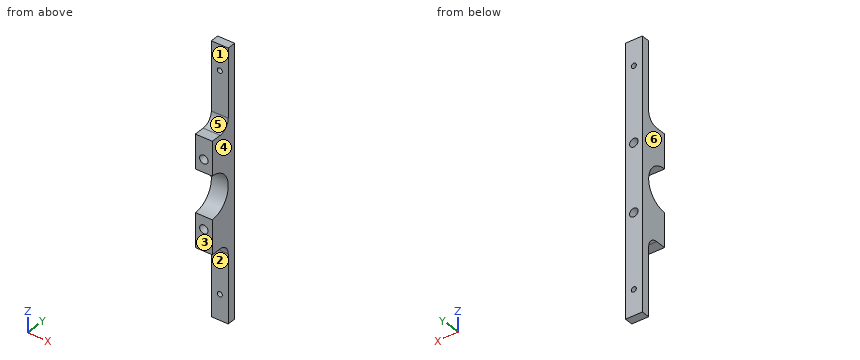
from build123d import *

# Parameters (mm, degrees)
BOSS_EXTRUDE1_DEPTH     = 10
CUT_EXTRUDE1_DEPTH      = 81.605520903
CUT_EXTRUDE1_DEPTH_BACK = 81.605520903
SKETCH2_R               = 1.5
SKETCH2_R_2             = 2.5
FILLET1_R               = 6.35


with BuildPart() as part:
    # Sketch1 → Boss-Extrude1 (new body)
    with BuildSketch(Plane(origin=(0, 0, 0), x_dir=(0, 0, -1), z_dir=(1, 0, 0))):
        with BuildLine():
            Line((-79, 12.5), (-32.5, 12.5))
            Line((-32.5, 12.5), (-32.5, 0))
            Line((-32.5, 0), (-12.5, 0))
            ThreePointArc((-12.5, 0), (0, 12.5), (12.5, 0))
            Line((12.5, 0), (32.5, 0))
            Line((32.5, 0), (32.5, 12.5))
            Line((32.5, 12.5), (79, 12.5))
            Line((79, 12.5), (79, 17.5))
            Line((79, 17.5), (-79, 17.5))
            Line((-79, 17.5), (-79, 12.5))
        make_face()
    extrude(amount=BOSS_EXTRUDE1_DEPTH)

    # Sketch2 → Cut-Extrude1 (cut, two sides: drawn at the far end of the back side and taken through both)
    with BuildSketch(Plane.XZ.offset(-12.5).offset(-CUT_EXTRUDE1_DEPTH_BACK)):
        with Locations(Location((5, 64, 0), (0, 0, 270))):
            Circle(SKETCH2_R)
        with Locations(Location((5, -64, 0), (0, 0, 90))):
            Circle(SKETCH2_R)
        with Locations(Location((5, 20, 0), (0, 0, 270))):
            Circle(SKETCH2_R_2)
        with Locations(Location((5, -20, 0), (0, 0, 90))):
            Circle(SKETCH2_R_2)
    extrude(amount=CUT_EXTRUDE1_DEPTH + CUT_EXTRUDE1_DEPTH_BACK, mode=Mode.SUBTRACT)

    # Fillet1
    fillet1_edges = [part.edges().sort_by_distance(p)[0] for p in [
        (5, 12.5, 32.5),
        (5, 12.5, -32.5),
    ]]
    fillet(fillet1_edges, radius=FILLET1_R)


solid = part.part
Geometry check sheet. Reference: the model listing, model coordinates, mm. Face numbers are marked on the shaded views. A direction names the side the tool comes from. Coordinates: 2 decimals unless noted, no trailing zeros. Order: outer loops, then holes, each group sorted by start corner. A loop starts at its lowest first (then second) coordinate and runs counter-clockwise, first axis right, second up. Notation, with made-up numbers: (31, -19) -> (72, -19) arc R24 cw to (72, 10) -> close; hole circle Ø6 at (59.25, 27.25). An arc over 180 degrees is marked (long way). Use a Markdown table: item, result. Add a question column.
1. Cross-section at B-B (x = 5). Enter the section's corners in (y, z).
2. Cross-section at C-C (y = 7.75). Enter the section's corners in (x, z).
3. Go/stop test with flat-tipped pins: pin 1 Ø3 at (x, y) = (3, 3) entering from -Z; pin 2 Ø1.5 at (x, y) = (4, 8) entering from +Z; pin 3 Ø1 at (x, y) = (3.5, 9) entering from -Z. Record where each tip stops, or that it passes through.
4. Set-up check for the marked faces 1, 2 and 3: record each of +Z, -Z, +X, -X, +Y, -Y from which the full face is reachable in a straight line by a thin tool's end or side.
5. Material ranges on L1, parallel to X at y = 4.75, z = -20; L2, parallel to X at y = 15.5, z = -64; L3, parallel to Z at x = 7.25, y = 5.5, recorded low to high.
6. Cross-section at D-D (z = -20). Enter the section's corners in (x, y), and give its area (3 significant figures).
7. Cross-section at A-A (z = 64). Enter the section's corners in (x, y).
8. Mould release check, pull along X, two halves, no side actions. Record for the marked faces 4, 5 and 6: pulls with the +X half, pulls with the -X half, needs draft (parallel to the pull), parting line crosses it, or undercut.
Filled sheet:
| question | item | result |
|---|---|---|
| 1 | outline | (0, -32.5) -> (6.15, -32.5) arc R6.35 cw to (12.5, -38.85) -> (12.5, -62.5) -> (17.5, -62.5) -> (17.5, -22.5) -> (0, -22.5) -> close; (0, -17.5) -> (17.5, -17.5) -> (17.5, 17.5) -> (0, 17.5) -> (0, 12.5) arc R12.5 cw to (0, -12.5) -> close; (0, 22.5) -> (17.5, 22.5) -> (17.5, 62.5) -> (12.5, 62.5) -> (12.5, 38.85) arc R6.35 cw to (6.15, 32.5) -> (0, 32.5) -> close; (12.5, -79) -> (17.5, -79) -> (17.5, -65.5) -> (12.5, -65.5) -> close; (12.5, 65.5) -> (17.5, 65.5) -> (17.5, 79) -> (12.5, 79) -> close |
| 2 | outline | (0, -32.7) -> (10, -32.7) -> (10, -9.81) -> (0, -9.81) -> close; (0, 9.81) -> (10, 9.81) -> (10, 32.7) -> (0, 32.7) -> close; hole circle Ø5 at (5, -20); hole circle Ø5 at (5, 20) |
| 3 | pin 1 | z = -32.5 |
| 3 | pin 2 | z = 33.06 |
| 3 | pin 3 | z = -33.46 |
| 4 | face 1 | +Z, +X, -X, -Y |
| 4 | face 2 | -Z, +X, -X, -Y |
| 4 | face 3 | +Z, -Z, +X, -X, -Y |
| 5 | L1 | 0 to 2.5, 7.5 to 10 |
| 5 | L2 | 0 to 3.5, 6.5 to 10 |
| 5 | L3 | -32.5 to -21.09, -18.91 to -11.22, 11.22 to 18.91, 21.09 to 32.5 |
| 6 | outline | (0, 0) -> (2.5, 0) -> (2.5, 17.5) -> (0, 17.5) -> close; (7.5, 0) -> (10, 0) -> (10, 17.5) -> (7.5, 17.5) -> close |
| 6 | area | 87.5 mm2 |
| 7 | outline | (0, 12.5) -> (3.5, 12.5) -> (3.5, 17.5) -> (0, 17.5) -> close; (6.5, 12.5) -> (10, 12.5) -> (10, 17.5) -> (6.5, 17.5) -> close |
| 8 | face 4 | pulls with the +X half |
| 8 | face 5 | needs draft |
| 8 | face 6 | pulls with the -X half |
